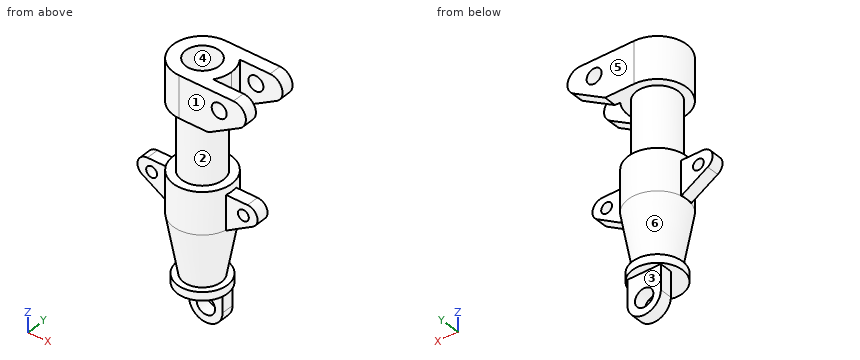
```python
from build123d import *

# Parameters (mm, degrees)
SKETCH2_R                = 6.5
SKETCH2_W                = 10
SKETCH2_H                = 41.021116242
BOSS_EXTRUDE1_DEPTH      = 7.5
SKETCH3_R                = 9
BOSS_EXTRUDE2_DEPTH      = 35
BOSS_EXTRUDE2_DEPTH_BACK = 35
BOSS_EXTRUDE3_START      = -10.090847
SKETCH4_W                = 24.58727528
SKETCH4_H                = 50
BOSS_EXTRUDE3_DEPTH      = 10.090847
CUT_EXTRUDE1_DEPTH       = 51
SKETCH6_R                = 11
BOSS_EXTRUDE4_DEPTH      = 20
SKETCH6_3_R              = 11
CUT_EXTRUDE2_DEPTH       = 5


with BuildPart() as part:
    # Sketch1 → Revolve1 (revolve)
    with BuildSketch(Plane(origin=(0, 0, 0), x_dir=(1, 0, 0), z_dir=(0, 1, 0))):
        Polygon((-35, 0), (-20, 0), (-20, 235), (0, 235), (0, 260), (-30, 260), (-30, 250), (-22.65711135, 250), (-35, 180), (-35, 130), (-25, 130), (-25, 50), (-35, 50), align=None)
    revolve(axis=Axis((0, 0, 0), (0, 0, -1)))

    # Sketch2 → Boss-Extrude1 (add, symmetric)
    with BuildSketch(Plane(origin=(0, 0, 0), x_dir=(1, 0, 0), z_dir=(0, 1, 0))):
        with BuildLine():
            ThreePointArc((-60, 138.978883758), (-71.563565439, 147.772023245), (-66.180456899, 161.264891366))
            Line((-66.180456899, 161.264891366), (-35, 180))
            Line((-35, 180), (-35, 138.978883758))
            Line((-35, 138.978883758), (-60, 138.978883758))
        make_face()
        with Locations((-55, 153.268883758)):
            Circle(SKETCH2_R, mode=Mode.SUBTRACT)
        with Locations((-30, 159.489441879)):
            Rectangle(SKETCH2_W, SKETCH2_H)
        with Locations((30, 159.489441879)):
            Rectangle(SKETCH2_W, SKETCH2_H)
        with BuildLine():
            Line((35, 138.978883758), (60, 138.978883758))
            ThreePointArc((60, 138.978883758), (71.563565439, 147.772023245), (66.180456899, 161.264891366))
            Line((66.180456899, 161.264891366), (35, 180))
            Line((35, 180), (35, 138.978883758))
        make_face()
        with Locations((55, 153.268883758)):
            Circle(SKETCH2_R, mode=Mode.SUBTRACT)
    extrude(amount=BOSS_EXTRUDE1_DEPTH, both=True)

    # Sketch3 → Boss-Extrude2 (add, two sides)
    with BuildSketch(Plane(origin=(0, 0, 0), x_dir=(1, 0, 0), z_dir=(0, 1, 0))) as boss_extrude2_sk:
        with BuildLine():
            Line((35, 0), (65, 0))
            ThreePointArc((65, 0), (79.474933129, 11.066005733), (72.592573861, 27.93649188))
            Line((72.592573861, 27.93649188), (35, 50))
            Line((35, 50), (24.58727528, 50))
            Line((24.58727528, 50), (24.58727528, 0))
            Line((24.58727528, 0), (35, 0))
        make_face()
        with Locations((48, 19)):
            Circle(SKETCH3_R, mode=Mode.SUBTRACT)
    extrude(amount=BOSS_EXTRUDE2_DEPTH)
    extrude(boss_extrude2_sk.sketch, amount=-BOSS_EXTRUDE2_DEPTH_BACK)

    # Sketch4 → Boss-Extrude3 (add)
    with BuildSketch(Plane(origin=(0, 35, 0), x_dir=(1, 0, 0), z_dir=(0, 1, 0)).offset(BOSS_EXTRUDE3_START)):
        with Locations((12.29363764, 25)):
            Rectangle(SKETCH4_W, SKETCH4_H)
    boss_extrude3 = extrude(amount=BOSS_EXTRUDE3_DEPTH)

    # Mirror1: Boss-Extrude3 across plane
    add(boss_extrude3.mirror(Plane.ZX))

    # Sketch5 → Cut-Extrude1 (cut, through all)
    with BuildSketch(Plane(origin=(0, 0, -50), x_dir=(-1, 0, 0), z_dir=(0, 0, -1))):
        Polygon((-90.173846019, 20), (-90.173846019, -20), (-35, -20), (-35, -3.8e-08), (-35, 20), align=None)
        with BuildLine():
            Line((-35, 20), (-35, -3.8e-08))
            ThreePointArc((-35, -3.8e-08), (-33.393850212, 10.480971713), (-28.722813233, 20))
            Line((-28.722813233, 20), (-35, 20))
        make_face()
        with BuildLine():
            Line((-35, -3.8e-08), (-35, -20))
            Line((-35, -20), (-28.722813233, -20))
            ThreePointArc((-28.722813233, -20), (-33.3938502, -10.480971749), (-35, -3.8e-08))
        make_face()
    extrude(amount=-CUT_EXTRUDE1_DEPTH, mode=Mode.SUBTRACT)

    # Sketch6 → Boss-Extrude4 (add)
    with BuildSketch(Plane(origin=(0, 0, 0), x_dir=(0, 0, -1), z_dir=(0, 1, 0))):
        with BuildLine():
            Line((260, 20), (260, -20))
            Line((260, -20), (290, -20))
            ThreePointArc((290, -20), (310, 0), (290, 20))
            Line((290, 20), (260, 20))
        make_face()
        with Locations((290, 0)):
            Circle(SKETCH6_R, mode=Mode.SUBTRACT)
    extrude(amount=BOSS_EXTRUDE4_DEPTH)

    # Sketch6<3> → Cut-Extrude2 (cut)
    with BuildSketch(Plane(origin=(0, 0, 0), x_dir=(0, 0, -1), z_dir=(0, 1, 0))):
        with BuildLine():
            Line((260, 20), (260, -20))
            Line((260, -20), (290, -20))
            ThreePointArc((290, -20), (310, 0), (290, 20))
            Line((290, 20), (260, 20))
        make_face()
        with Locations((290, 0)):
            Circle(SKETCH6_3_R, mode=Mode.SUBTRACT)
    extrude(amount=CUT_EXTRUDE2_DEPTH, mode=Mode.SUBTRACT)


solid = part.part
```
Geometry check sheet. Reference: the model listing, model coordinates, mm. Face numbers are marked on the shaded views. A direction names the side the tool comes from. Coordinates: 2 decimals unless noted, no trailing zeros. Order: outer loops, then holes, each group sorted by start corner. A loop starts at its lowest first (then second) coordinate and runs counter-clockwise, first axis right, second up.
Q1. Tool access check on the marked faces 1, 2 and 3. Record the directions out of +Z, -Z, +X, -X, +Y, -Y that give a thin tool (end or side, any length) a straight path to the whole face; none if there is none.
Reply:
face 1: +Z, -Z, +X, -X, -Y
face 2: none
face 3: -Z, +X, -X, +Y
Q2. Sectioned sample at A-A on z = -19. Record the cut outline in (x, y).
Reply:
outline: (0, -35) - (39, -35) - (39, -20) - (28.72, -20) arc R35 ccw to (28.72, 20) - (39, 20) - (39, 35) - (0, 35) arc R35 ccw to start; (57, -35) - (79.46, -35) - (79.46, -20) - (57, -20) - close; (57, 20) - (79.46, 20) - (79.46, 35) - (57, 35) - close; hole circle Ø40 at (0, 0)
Q3. Thickness scan on probe 1 along Y at (x, z) = (0, -94); probe 2 along Z at (x, y) = (0, 9); probe 3 along X at (y, z) = (8, -290). Record the ranges inside material, lowest first.
Reply:
probe 1: y = -25 to -20, 20 to 25
probe 2: z = -310 to -301, -279 to -235
probe 3: x = -20 to -11, 11 to 20
Q4. Depth check by flat-ended pin: pin 1 Ø4 at (x, y) = (-13.5, -4.5) entering from +Z; pin 2 Ø3 at (x, y) = (-6, 1.5) entering from -Z; pin 3 Ø12 at (x, y) = (42.5, 13) entering from +Z. Enter the tip coordinate at first touch or a pass-through.
Reply:
pin 1: stops at z = -235
pin 2: stops at z = -260
pin 3: stops at z = -138.98
Q5. Sectioned sample at C-C on x = 44. Record the cut outline in (y, z).
Reply:
outline: (-35, -44.72) - (-20, -44.72) - (-20, -27.06) - (-35, -27.06) - close; (-35, -10.94) - (-20, -10.94) - (-20, 0) - (-35, 0) - close; (-7.5, -174.59) - (7.5, -174.59) - (7.5, -138.98) - (-7.5, -138.98) - close; (20, -44.72) - (35, -44.72) - (35, -27.06) - (20, -27.06) - close; (20, -10.94) - (35, -10.94) - (35, 0) - (20, 0) - close
Q6. Sectioned sample at D-D on z = -167. Record the cut outline in (x, y).
Reply:
outline: (-56.64, -7.5) - (-34.19, -7.5) arc R35 ccw to (34.19, -7.5) - (56.64, -7.5) - (56.64, 7.5) - (34.19, 7.5) arc R35 ccw to (-34.19, 7.5) - (-56.64, 7.5) - close; hole circle Ø40 at (0, 0)
Q7. Sectioned sample at B-B on x = -55. Record the cut outline in (y, z), and give its area (3 significant figures).
Reply:
outline: (-7.5, -167.98) - (7.5, -167.98) - (7.5, -159.77) - (-7.5, -159.77) - close; (-7.5, -146.77) - (7.5, -146.77) - (7.5, -138.98) - (-7.5, -138.98) - close
area: 240 mm2
Q8. Draft check along Y on the marked faces 4, 5 and 6. Enter one of: released by +Y, released by -Y, zero draft, split by the parting line, or undercut.
Reply:
face 4: undercut
face 5: released by +Y
face 6: split by the parting line
